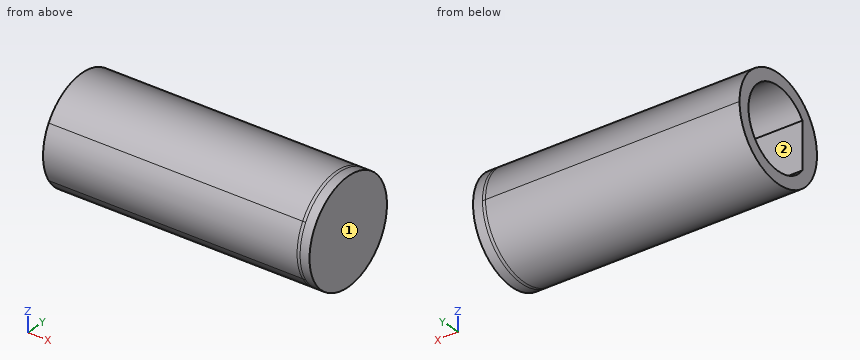
from build123d import *

# Parameters (mm, degrees)
BOSS_EXTRUDE1_START = 0.2
BOSS_EXTRUDE1_DEPTH = 17
BOSS_EXTRUDE2_START = 0.825
SKETCH1_3_R         = 3.45
BOSS_EXTRUDE2_DEPTH = 0.825


with BuildPart() as part:
    # Sketch1 → Boss-Extrude1 (new body)
    # profile 1 of 2: a face of its own
    with BuildSketch(Plane(origin=(7.999998093, 0, 0), x_dir=(0, 0, -1), z_dir=(1, 0, 0)).offset(BOSS_EXTRUDE1_START)):
        with BuildLine():
            Line((23.853743883, -20.744040957), (20.276035119, -20.744040824))
            ThreePointArc((20.276035119, -20.744040824), (18.742240101, -16.865331986), (22.06488974, -14.344040891))
            ThreePointArc((22.06488974, -14.344040891), (25.387539191, -16.865332234), (23.853743883, -20.744040957))
        make_face()
        with BuildLine():
            ThreePointArc((23.61408287, -19.944040948), (24.586793684, -16.980099955), (22.06488971, -15.144040891))
            ThreePointArc((22.06488971, -15.144040891), (19.542985599, -16.980099767), (20.515696193, -19.944040833))
            Line((20.515696193, -19.944040833), (23.61408287, -19.944040948))
        make_face(mode=Mode.SUBTRACT)
    # profile 2 of 2: a face of its own
    with BuildSketch(Plane(origin=(7.999998093, 0, 0), x_dir=(0, 0, -1), z_dir=(1, 0, 0)).offset(BOSS_EXTRUDE1_START)):
        with BuildLine():
            ThreePointArc((20.276035119, -20.744040824), (22.064889483, -21.244040891), (23.853743883, -20.744040957))
            Line((23.853743883, -20.744040957), (20.276035119, -20.744040824))
        make_face()
    extrude(amount=-BOSS_EXTRUDE1_DEPTH)

    # Sketch1<3> → Boss-Extrude2 (add)
    with BuildSketch(Plane(origin=(7.999998093, 0, 0), x_dir=(0, 0, -1), z_dir=(1, 0, 0)).offset(BOSS_EXTRUDE2_START)):
        with Locations(Location((22.064889611, -17.794040891, 0), (0, 0, 90))):
            Circle(SKETCH1_3_R)
        with BuildLine():
            Line((23.853743883, -20.744040957), (20.276035119, -20.744040824))
            ThreePointArc((20.276035119, -20.744040824), (18.742240101, -16.865331986), (22.06488974, -14.344040891))
            ThreePointArc((22.06488974, -14.344040891), (25.387539191, -16.865332234), (23.853743883, -20.744040957))
        make_face()
    extrude(amount=-BOSS_EXTRUDE2_DEPTH)


solid = part.part
Build history of the part. All positions in model axes, mm. Face numbers are marked on the shaded views. Give positions to 0.01 mm unless a question says otherwise; leave off trailing zeros. Order: outer loops, then holes, each group sorted by start corner. A loop starts at its lowest first (then second) coordinate and runs counter-clockwise, first axis right, second up. Notation, with made-up numbers: M 40.5,64 L 88.5,64 A22 ccw 88.5,87 Z; hole C -16,17.25 d6. An arc over 180 degrees is marked long. Put each result on its own line as item: value.
Item 1: Cut at C-C on z = -22.25. Write the cut outline in (x, y) (3 decimals), then the cut area to 3 significant figures.
Results are:
outline: M -8.8,-21.239 L 8.825,-21.239 L 8.825,-14.349 L -8.8,-14.349 L -8.8,-15.151 L 8,-15.151 L 8,-19.944 L -8.8,-19.944 Z
area: 40.9 mm2
Item 2: Cut at A-A on x = 4. Write the cut outline in (y, z).
Results are:
outline: C -17.79,-22.06 d6.9; hole M -19.94,-23.61 A2.65 ccw long -19.94,-20.52 Z
Item 3: Cut at B-B on y = -18. Write the cut outline in (x, z) (3 decimals), then the cut area to 3 significant figures.
Results are:
outline: M -8.8,-25.509 L 8.825,-25.509 L 8.825,-18.621 L -8.8,-18.621 L -8.8,-19.423 L 8,-19.423 L 8,-24.707 L -8.8,-24.707 Z
area: 32.6 mm2
Item 4: Pull direction Y, two halves, no side cores. Call the marked faces 1 and 2: +Y half, -Y half, draft (parallel to the pull), parting line (faces both ways), or undercut.
Results are:
face 1: draft
face 2: undercut
Item 5: Wall check: probe 1 along Z at (x, y) = (6.5, -17.75); probe 2 along X at (y, z) = (-19.5, -23.5) (3 decimals); probe 3 along Z at (x, y) = (-2.25, -19.75). Give the ranges that are in metal, low to high.
Results are:
probe 1: -25.51 to -24.71, -19.42 to -18.62
probe 2: 8 to 8.825
probe 3: -24.91 to -23.85, -20.28 to -19.22
Item 6: Cut at D-D on y = -20.25. Write the cut outline in (x, z) (3 decimals), then the cut area to 3 significant figures.
Results are:
outline: M -8.8,-24.488 L 8.825,-24.488 L 8.825,-19.642 L -8.8,-19.642 Z
area: 85.4 mm2
Item 7: Drop flat-ended pins along their axis: pin 1 Ø3.5 at (x, z) = (3.5, -22.5) entering from +Y; pin 2 Ø1.5 at (x, y) = (4.5, -19) entering from +Z; pin 3 Ø1 at (x, y) = (-6, -15.5) entering from +Z; pin 4 Ø1 at (x, y) = (1, -19) entering from +Z. Give the stop position or say it passes through.
Results are:
pin 1: y = -14.34
pin 2: z = -18.65
pin 3: z = -19.12
pin 4: z = -18.69
